```python
from build123d import *

# Parameters (mm, degrees)
SKETCH_1_W          = 35
SKETCH_1_H          = 70
EXTRUDE_1_DEPTH     = 12
CUT_EXTRUDE_1_REACH = 81.177


with BuildPart() as part:
    # 草图1 → 凸台-拉伸1 (new body)
    with BuildSketch(Plane.XY):
        with Locations((17.5, -35)):
            Rectangle(SKETCH_1_W, SKETCH_1_H)
    extrude(amount=EXTRUDE_1_DEPTH)

    # 草图2 → 切除-拉伸1 (cut, up to next)
    with BuildSketch(Plane.XZ.offset(70), mode=Mode.PRIVATE) as cut_extrude_1_sk1:
        Polygon((10, 12), (10, 11.5), (6.5, 7.328862426), (6.5, 5), (35, 5), (35, 12), align=None)
    cut_extrude_1_tool1 = extrude(cut_extrude_1_sk1.sketch, amount=-CUT_EXTRUDE_1_REACH, mode=Mode.PRIVATE) & part.part
    add(cut_extrude_1_tool1.solids().sort_by_distance((21.366311, -70, 8.408444))[0], mode=Mode.SUBTRACT)


solid = part.part
```
For this review, take the finished solid that the model builds, in its own axes (mm). Round coordinates to 2 decimals unless told otherwise and drop trailing zeros. Write each loop counter-clockwise with the first axis right and the second up, starting at its lowest first coordinate (ties: lowest second). Pieces come first, ordered by that corner, then holes. Notation, with made-up numbers: M 52.5,5 L 69.5,5 A14 cw 69.5,15 Z; hole C 34.25,4 d10. An arc over 180 degrees is marked long. One line per item, written item: value. Start each with the question number.
(1) We need section B-B (x = 32). Give the boundary of the cut face in (y, z), and give its area (3 significant figures).
(2) We need section C-C (z = 8.5). Give the boundary of the cut face in (x, y).
(3) Wall thickness on line 1 (Z direction, x = 22.5, y = -37.5); line 2 (X direction, y = -12, z = 11.75); line 3 (Z direction, x = 9, y = -56): over which ranges is each line inside the solid? List them lowest first.
(4) We need section A-A (y = -59). Give the boundary of the cut face in (x, z), and give its area (3 significant figures).
(5) The part is to be moulded in two halves that separate along Z. For faces 1 (the flat face through (6.5, -35, 6)), 2 (the flat face through (17, -35, 0)), 3 (the flat face through (8.27, -35.49, 9.44)), 4 (the flat face through (0, -35, 6)), say which applies: released by +Z, released by -Z, zero draft, split by the parting line, or undercut.
(6) Insertion check: pin 1 (5 mm diameter, centred on x = 15.5, y = -57, fed in from -Z); pin 2 (10 mm diameter, centred on x = 23.5, y = -13.5, fed in from +Z). Each pin has a flat end and moves straight along its axis. Give the tip position at first contact, or say it passes through.
Result:
1. outline: M -70,0 L 0,0 L 0,5 L -70,5 Z
1. area: 350 mm²
2. outline: M 0,-70 L 7.48,-70 L 7.48,0 L 0,0 Z
3. line 1: 0 to 5
3. line 2: 0 to 10
3. line 3: 0 to 5, 10.31 to 12
4. outline: M 0,0 L 35,0 L 35,5 L 6.5,5 L 6.5,7.33 L 10,11.5 L 10,12 L 0,12 Z
4. area: 230 mm²
5. face 1: undercut
5. face 2: released by -Z
5. face 3: undercut
5. face 4: zero draft
6. pin 1: z = 0
6. pin 2: z = 5
